Could you check a few things on this drawing? It's one solid part, dimensions in mm from its lowest x, y, z. Give positions to 0.01 mm unless a question says otherwise; leave off trailing zeros. Loops run counter-clockwise (first coordinate to the right, second up) from the corner with the lowest first, then second, coordinate; pieces in that order, holes last. Notation, with made-up numbers: (-31.5, 15.25) - (-14.5, 15.25) arc R25 ccw to (-14.5, 46.25) - close; hole circle Ø2 at (-4.75, -39). An arc over 180 degrees is marked (long way). Write item = value, one per line.
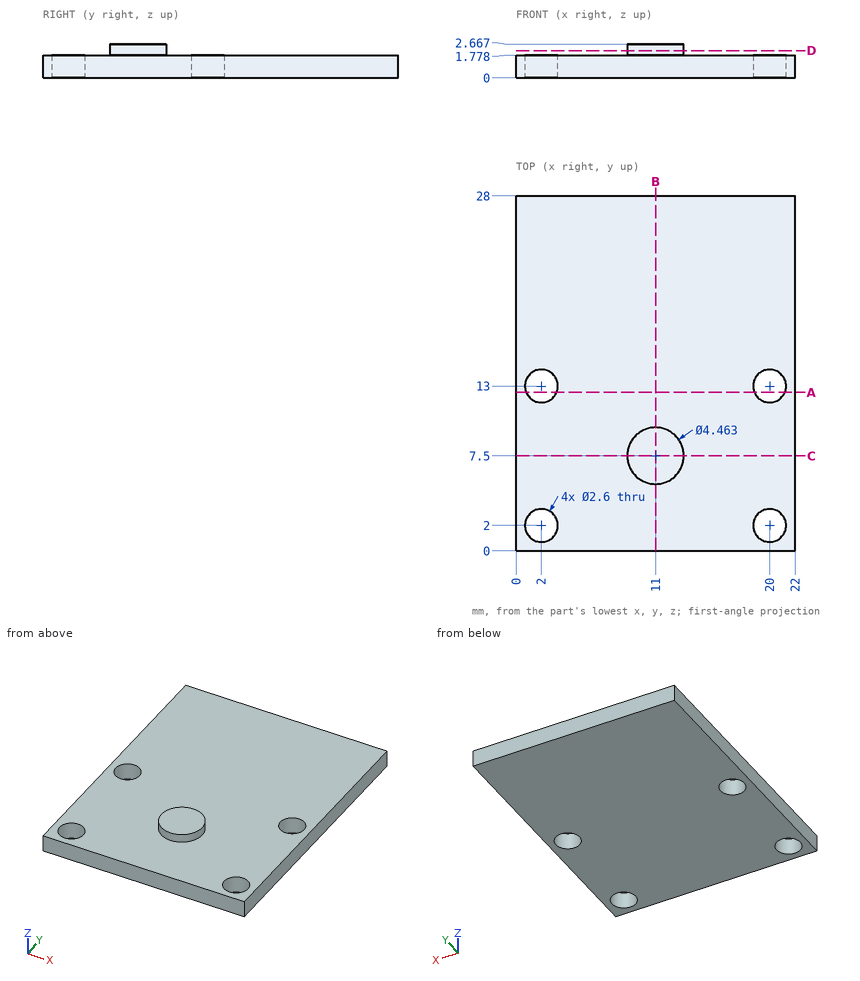
Q1. Imagine slicing it at C-C, the plane y = 7.5. Write out the boundary of the cut face in (x, z).
Output:
outline = (0, 0) - (22, 0) - (22, 1.78) - (13.23, 1.78) - (13.23, 2.67) - (8.77, 2.67) - (8.77, 1.78) - (0, 1.78) - close
Q2. For pin 1 (3 mm diameter, centred on x = 13.5, y = 20, fed in from +Z), with a flat end and sliding along its axis, tell me the tip position at first contact or that it passes through.
Output:
pin_1 = 1.78
Q3. I need wall thicknesses on L1, parallel to Y at x = 2, z = 0.65; L2, parallel to Z at x = 10.25, y = 25.25. Which ranges of each line are inside material? Lowest first, please.
Output:
L1 = 0 to 0.7, 3.3 to 11.7, 14.3 to 28
L2 = 0 to 1.78
Q4. Imagine slicing it at A-A, the plane y = 12.5. Write out the boundary of the cut face in (x, z).
Output:
outline = (0, 0) - (0.8, 0) - (0.8, 1.78) - (0, 1.78) - close; (3.2, 0) - (18.8, 0) - (18.8, 1.78) - (3.2, 1.78) - close; (21.2, 0) - (22, 0) - (22, 1.78) - (21.2, 1.78) - close
Q5. Imagine slicing it at D-D, the plane z = 2.15. Write out the boundary of the cut face in (x, y).
Output:
outline = circle Ø4.46 at (11, 7.5)
Q6. Imagine slicing it at B-B, the plane x = 11. Write out the boundary of the cut face in (y, z).
Output:
outline = (0, 0) - (28, 0) - (28, 1.78) - (9.73, 1.78) - (9.73, 2.67) - (5.27, 2.67) - (5.27, 1.78) - (0, 1.78) - close
